from build123d import *

# Parameters (mm, degrees)
EXTRUDE_1_DEPTH     = 27
FILLET_1_R          = 1.5
FILLET_2_R          = 1.5
CUT_EXTRUDE_1_DEPTH = 27
CUT_EXTRUDE_2_DEPTH = 27
SKETCH_5_W          = 21
SKETCH_5_H          = 23
CUT_EXTRUDE_3_DEPTH = 27


with BuildPart() as part:
    # 草图1 → 凸台-拉伸1 (new body)
    with BuildSketch(Plane.XY):
        Polygon((-11.5, 11.5), (11.5, -11.5), (17.5, -11.5), (17.5, -17.5), (-17.5, -17.5), (-17.5, 17.5), (-11.5, 17.5), align=None)
    extrude(amount=EXTRUDE_1_DEPTH)

    # 圆角1
    fillet_1_edges = [part.edges().sort_by_distance(p)[0] for p in [
        (-11.5, 17.5, 13.5),
        (17.5, -11.5, 13.5),
    ]]
    fillet(fillet_1_edges, radius=FILLET_1_R)

    # 圆角2
    fillet_2_edges = [part.edges().sort_by_distance(p)[0] for p in [
        (-17.5, -17.5, 13.5),
        (-17.5, 0, 27),
        (0, -17.5, 27),
        (0, -17.5, 0),
        (-17.5, 0, 0),
    ]]
    fillet(fillet_2_edges, radius=FILLET_2_R)

    # 草图2 → 切除-拉伸1 (cut)
    with BuildSketch(Plane.XZ.offset(17.5)):
        with BuildLine():
            Line((0, 16.550659992), (8, 16.550659992))
            ThreePointArc((8, 16.550659992), (11, 13.550659992), (8, 10.550659992))
            Line((8, 10.550659992), (0, 10.550659992))
            ThreePointArc((0, 10.550659992), (-3, 13.550659992), (0, 16.550659992))
        make_face()
    extrude(amount=-CUT_EXTRUDE_1_DEPTH, mode=Mode.SUBTRACT)

    # 草图3 → 切除-拉伸2 (cut)
    with BuildSketch(Plane.ZY.offset(17.5)):
        with BuildLine():
            Line((10.5, 0), (10.5, 8))
            ThreePointArc((10.5, 8), (13.5, 11), (16.5, 8))
            Line((16.5, 8), (16.5, 0))
            ThreePointArc((16.5, 0), (13.5, -3), (10.5, 0))
        make_face()
    extrude(amount=-CUT_EXTRUDE_2_DEPTH, mode=Mode.SUBTRACT)

    # 草图5 → 切除-拉伸3 (cut)
    with BuildSketch(Plane(origin=(11, 0, 0), x_dir=(0, 0, -1), z_dir=(1, 0, 0))):
        with Locations((-13.5, 0)):
            Rectangle(SKETCH_5_W, SKETCH_5_H)
    extrude(amount=-CUT_EXTRUDE_3_DEPTH, mode=Mode.SUBTRACT)


solid = part.part
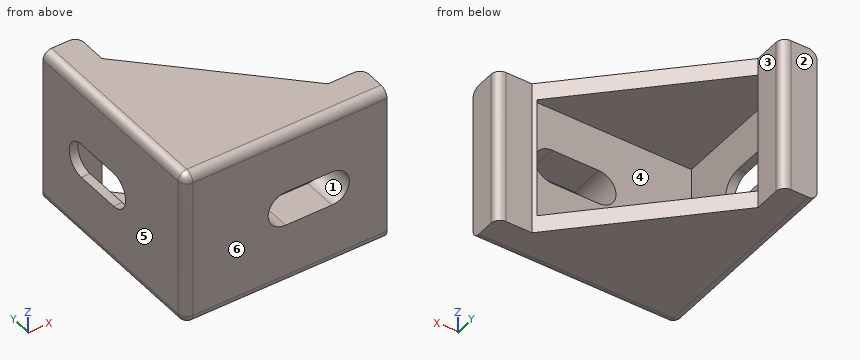
Source: CAD feature listing. Evaluate the final solid. Frame: model axes, mm. Face numbers are marked on the shaded views. A direction names the side the tool comes from. Coordinates: 2 decimals unless noted, no trailing zeros. Loops run counter-clockwise (first coordinate to the right, second up) from the corner with the lowest first, then second, coordinate; pieces in that order, holes last. Notation, with made-up numbers: (46.5, -13.75) -> (94.5, -13.75) arc R28 cw to (94.5, 11.25) -> close; hole circle Ø10 at (-33.5, 15.25). An arc over 180 degrees is marked (long way). Answer in a Markdown table with one row per item. Add a question column.
Q1. Ray query, line 1 along Y through (x, z) = (-15, 3.75); line 2 along Z through (x, y) = (-3, -4); line 3 along X through (y, z) = (1, 21.5). Return the intervals inside material, ascending.
Q2. Section C-C on z = 5. Return the cut outline in (x, y).
Q3. Section B-B on x = 10. Return the cut outline in (y, z).
Q4. Section A-A on y = -14. Return the cut outline in (x, z), and give its area (3 significant figures).
Q5. Contact query for flat-ended pins moving along their axis: pin 1 Ø0.8 at (x, y) = (-16.5, 3) entering from -Z; pin 2 Ø0.8 at (x, y) = (-17, 4.5) entering from +Z; pin 3 Ø10.5 at (x, z) = (1.5, 17) entering from +Y; pin 4 Ø3 at (x, y) = (2.5, 1.5) entering from -Z. Output: stop coordinate, or through.
Q6. Reachability of the marked faces 1, 2 and 3 from +Z, -Z, +X, -X, +Y, -Y: full face, straight path, thin tool, end or side. Return the list, or none.
Q7. Pull-direction query (Y, two-part tool) for the marked faces 4, 5 and 6; classes: pulls with the +Y half, pulls with the -Y half, needs draft (parallel to the pull), parting line crosses it, or undercut.
Q8. Section D-D on y = -0.5. Return the cut outline in (x, z).
Computed values:
| question | item | result |
|---|---|---|
| 1 | line 1 | y = -17.5 to -11.5, 11.5 to 17.5 |
| 1 | line 2 | z = 0 to 3, 24 to 27 |
| 1 | line 3 | x = -17.5 to -16 |
| 2 | outline | (-17.5, -16) arc R1.5 ccw to (-16, -17.5) -> (17.5, -17.5) -> (17.5, -13) arc R1.5 ccw to (16, -11.5) -> (11.5, -11.5) -> (11, -11) -> (11, -11.5) -> (-16, -11.5) -> (-16, 11.5) -> (-11.5, 11.5) -> (-11.5, 16) arc R1.5 ccw to (-13, 17.5) -> (-17.5, 17.5) -> close |
| 3 | outline | (-17.5, 1.5) arc R1.5 ccw to (-16, 0) -> (-10, 0) -> (-10, 3) -> (-11.5, 3) -> (-11.5, 11.31) -> (-17.5, 11.31) -> close; (-17.5, 15.79) -> (-11.5, 15.79) -> (-11.5, 24) -> (-10, 24) -> (-10, 27) -> (-16, 27) arc R1.5 ccw to (-17.5, 25.5) -> close |
| 4 | outline | (-17.5, 1.5) arc R1.5 ccw to (-16, 0) -> (17.5, 0) -> (17.5, 27) -> (-16, 27) arc R1.5 ccw to (-17.5, 25.5) -> close; hole (0, 10.55) -> (8, 10.55) arc R3 ccw to (8, 16.55) -> (0, 16.55) arc R3 ccw to start |
| 4 | area | 868 mm^2 |
| 5 | pin 1 | stops at z = 0 |
| 5 | pin 2 | stops at z = 26.87 |
| 5 | pin 3 | stops at y = -11.5 |
| 5 | pin 4 | passes through |
| 6 | face 1 | +Y, -Y |
| 6 | face 2 | +Z, -Z, +X, -X, +Y |
| 6 | face 3 | +Z, -Z, +X, +Y |
| 7 | face 4 | undercut |
| 7 | face 5 | needs draft |
| 7 | face 6 | pulls with the -Y half |
| 8 | outline | (-17.5, 1.5) arc R1.5 ccw to (-16, 0) -> (0.5, 0) -> (0.5, 3) -> (-16, 3) -> (-16, 10.54) -> (-17.5, 10.54) -> close; (-17.5, 16.46) -> (-16, 16.46) -> (-16, 24) -> (0.5, 24) -> (0.5, 27) -> (-16, 27) arc R1.5 ccw to (-17.5, 25.5) -> close |
